Autodesk Inventor part; units mm, degrees
ref_plane "YZ Plane" through (0, 0, 0) normal (1, 0, 0) x (0, 1, 0)
ref_plane "XZ Plane" through (0, 0, 0) normal (0, 1, 0) x (-1, 0, 0)
ref_plane "XY Plane" through (0, 0, 0) normal (0, 0, 1) x (1, 0, 0)
sketch "Skizze1" plane through (0, 0, 0) normal (0, 0, 1) x (1, 0, 0)
  arc A0 (-8.312, -5) -> (-8.8369, -4) centre (0, 0) ccw
  line L0 (-18.5, -7) -> (-8.4853, -7)
  line L1 (-18.5, -7) -> (-18.5, -5)
  line L2 (-18.5, -5) -> (-8.312, -5)
  line L3 (-18.5, -2) -> (-18.5, -4)
  line L4 (-18.5, -4) -> (-8.8369, -4)
  line L5 (-18.5, -2) -> (-14.8661, -2)
  arc A1 (-8.4853, -7) -> (-10.9018, 1.4667) centre (0, 0) ccw
  arc A2 (-14.8661, -2) -> (-10.9018, 1.4667) centre (-14.8661, 2) ccw
  point P0 (-10.8167, -2)
  dimension "d0" = 19.4
  dimension "d2" = 2
  dimension "d4" = 1
  dimension "d5" = 18.5
  dimension "d6" = 4
  dimension "d7" = 1.3
  dimension "d19" = 10.0147
  dimension "d27" = 4
  dimension "d28" = 3.6339
extrude "Extrusion1" add sketch "Skizze1" along normal mid plane 14
sketch "Skizze2" plane through (-18.5, -2, 7) normal (0, 1, 0) x (1, 0, 0)
  circle A0 centre (3, 11) radius 1.65
  line L0 (0, 14) -> (3.6339, 14)
  line L1 (0, 14) -> (0, 0)
  line L2 (0, 14) -> (0, 0) construction
  line L3 (0, 7) -> (7.2294, 7) construction
  circle A1 centre (3, 3) radius 1.65
  circle A2 centre (3, 11) radius 3
  circle A3 centre (3, 3) radius 3
  point P0 (18.5, 7)
  point P1 (9.7894, 16)
  point P2 (0, 3)
  point P3 (0, 1.3417)
  point P4 (1.1676, 16)
  point P5 (0, 11)
  point P6 (0, 11.3417)
  point P7 (3, 14)
  dimension "d10" = 3
  dimension "d12" = 3.3
  dimension "d20" = 6
  dimension "d29" = 3
extrude "Extrusion2" cut sketch "Skizze2" against normal through all both and the other way through all contours A0 | A1
fillet "Rundung2" radius 4 1 edges at (-8.4853, -7, 0)
fillet "Rundung3" radius 0.8 2 edges at (-8.8369, -4, 0) (-8.312, -5, 0)
extrude "Extrusion4" cut sketch "Skizze2" along normal blind 10 contours A3 | A2
properties part number "Halterung_Pumpe_210403"
Input: part model. Units: mm. Frame: model coordinates. A direction names the side the tool comes from. Give positions to 0.01 mm unless a question says otherwise; leave off trailing zeros. Order: outer loops, then holes, each group sorted by start corner. A loop starts at its lowest first (then second) coordinate and runs counter-clockwise, first axis right, second up. Notation, with made-up numbers: (71, -28.75) -> (80, -28.75) arc R26 cw to (80, -10.75) -> close; hole circle Ø10 at (84.5, -32). An arc over 180 degrees is marked (long way). Write each question's results on one line, items separated by ' | '. Start each with the question number.
Item 1: Set-up query: faces 1 (the cylindrical face through (-9.348, -3.663, -0.098)), 2 (the flat face through (-16, -2, 0)), 3 (the flat face through (-14, -5, 0)). Return all of +Z, -Z, +X, -X, +Y, -Y with unobstructed straight access to the full face (end or side cutting, diameter ignored); none if empty.
Item 2: Cut plane C-C on y = 8.5. Return the cut outline in (x, z), then the cut area to 3 significant figures.
Item 3: Cut plane B-B on y = -6.25. Return the cut outline in (x, z).
Item 4: Cut plane A-A on x = -15.5. Return the cut outline in (y, z), then the cut area to 3 significant figures.
Item 5: Line query: line 1 (Z direction, x = -15.5, y = -3.05); line 2 (Y direction, x = -16.5, z = 1.5); line 3 (X direction, y = -5.85, z = -4). Output: solid intervals per line, ascending.
Item 6: Contact query for flat-ended pins moving along their axis: P1, Ø2.5, axis at x = -13, z = -1, coming from the -Y side; P2, Ø5.5, axis at x = -15.5, z = 4, coming from the +Y side; P3, Ø4, axis at x = -11, z = 1, coming from the +Y side. Output: stop coordinate, or through.
Item 7: Mould query, pull axis X, two halves, no side actions, for faces 4 (the cylindrical face through (-11.76, -0.52, -0.1)), 5 (the cylindrical face through (8.56, 4.56, -0.1)), 6 (the flat face through (-14, -4, 0)). Classes: pulls with the +X half, pulls with the -X half, needs draft (parallel to the pull), parting line crosses it, or undercut.
Item 8: Cut plane D-D on z = 0.25. Return the cut outline in (x, y).
Established:
1) face 1: +Z, -Z | face 2: -X, +Y | face 3: +Z, -Z, -X
2) outline: (-6.98, -7) -> (-4.67, -7) -> (-4.67, 7) -> (-6.98, 7) -> close; (4.67, -7) -> (6.98, -7) -> (6.98, 7) -> (4.67, 7) -> close | area: 64.6 mm^2
3) outline: (-18.5, -7) -> (-7.42, -7) -> (-7.42, 7) -> (-18.5, 7) -> close; (7.42, -7) -> (9.05, -7) -> (9.05, 7) -> (7.42, 7) -> close; hole circle Ø3.3 at (-15.5, -4); hole circle Ø3.3 at (-15.5, 4)
4) outline: (-7, -7) -> (-5, -7) -> (-5, -5.65) -> (-7, -5.65) -> close; (-7, -2.35) -> (-5, -2.35) -> (-5, 2.35) -> (-7, 2.35) -> close; (-7, 5.65) -> (-5, 5.65) -> (-5, 7) -> (-7, 7) -> close; (-4, -7) -> (-2, -7) -> (-2, -5.65) -> (-4, -5.65) -> close; (-4, -2.35) -> (-2, -2.35) -> (-2, 2.35) -> (-4, 2.35) -> close; (-4, 5.65) -> (-2, 5.65) -> (-2, 7) -> (-4, 7) -> close | area: 29.6 mm^2
5) line 1: -7 to -5.65, -2.35 to 2.35, 5.65 to 7 | line 2: -7 to -5, -4 to -2 | line 3: -18.5 to -17.15, -13.85 to -7.74, 7.74 to 9.32
6) P1: y = -7 | P2: y = -2 | P3: y = 6.32
7) face 4: pulls with the -X half | face 5: undercut | face 6: needs draft
8) outline: (-18.5, -7) -> (-10.2, -7) arc R4 cw to (-7.48, -8.07) arc R11 ccw (long way) to (-10.9, 1.47) arc R4 cw to (-14.87, -2) -> (-18.5, -2) -> (-18.5, -4) -> (-10, -4) arc R0.8 ccw to (-9.24, -2.96) arc R9.7 cw (long way) to (-8.09, -5.36) arc R0.8 ccw to (-8.75, -5) -> (-18.5, -5) -> close
